For this review, use the dimensioned drawing (mm, ordinates from the lowest corner) and the shaded views. A direction names the side the tool comes from. Give positions to 0.01 mm unless a question says otherwise; leave off trailing zeros. Write each loop counter-clockwise with the first axis right and the second up, starting at its lowest first coordinate (ties: lowest second). Pieces come first, ordered by that corner, then holes. Notation, with made-up numbers: (61.5, 20.5) -> (70.5, 20.5) arc R22 cw to (70.5, 46.5) -> close; hole circle Ø11 at (-10.5, -32). An arc over 180 degrees is marked (long way). Answer as CSV lines item,"result".
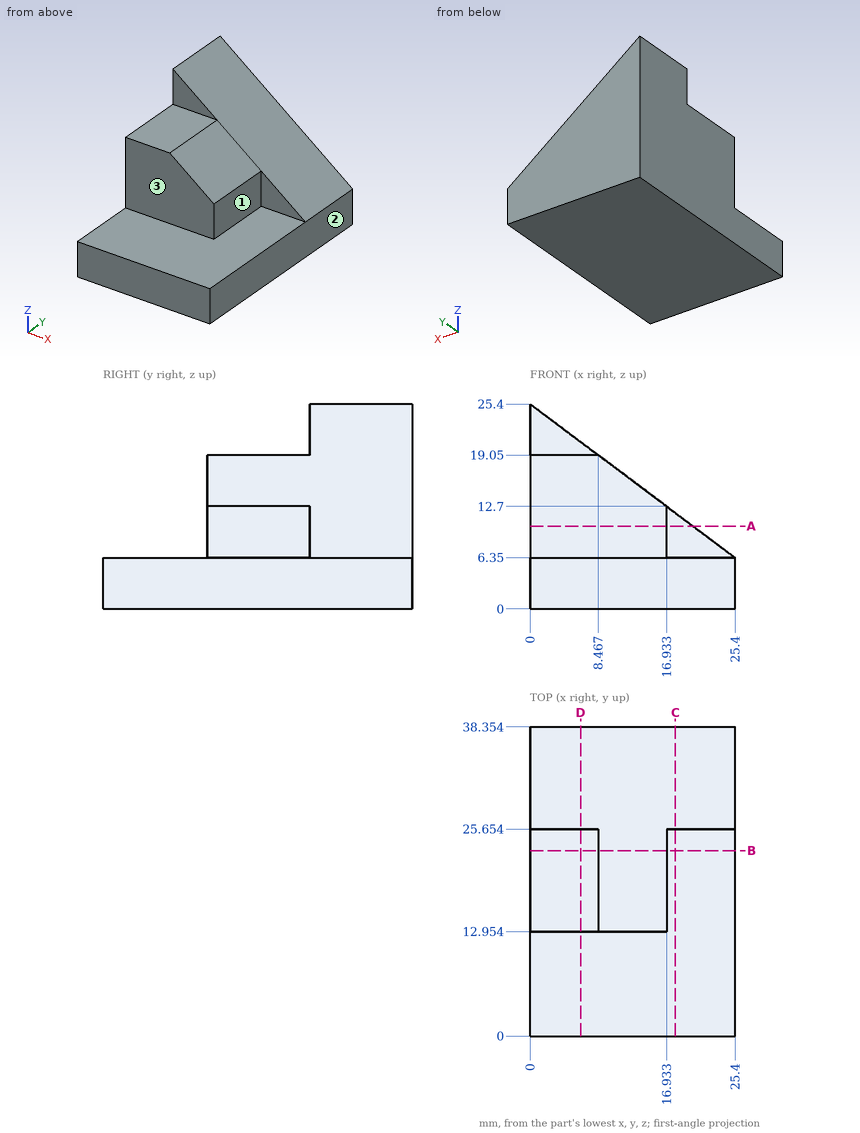
Q1. Add section A-A (z = 10.25). Write out the cut boundary in (x, y), plus the area to 3 significant figures.
Answer block:
outline,"(0, 12.95) -> (16.93, 12.95) -> (16.93, 25.65) -> (20.2, 25.65) -> (20.2, 38.35) -> (0, 38.35) -> close"
area,"472 mm2"
Q2. Add section B-B (y = 23). Write out the cut boundary in (x, z).
Answer block:
outline,"(0, 0) -> (25.4, 0) -> (25.4, 6.35) -> (16.93, 6.35) -> (16.93, 12.7) -> (8.47, 19.05) -> (0, 19.05) -> close"
Q3. To check wall thickness, follow probe 1 along Z at (x, y) = (15.75, 11.5); probe 2 along Y at (x, z) = (1, 23.5); probe 3 along Y at (x, z) = (4.25, 6.5). State the ranges of each line that lie inside material, in increasing order. Write a range as [from, to].
Answer block:
probe 1,"z = [0, 6.35]"
probe 2,"y = [25.65, 38.35]"
probe 3,"y = [12.95, 38.35]"
Q4. For the marked faces 1, 2 and 3, list the 3-axis set-ups (+Z, -Z, +X, -X, +Y, -Y) from which the entire face can be reached by the end or side of a thin tool; tool diameter is ignored.
Answer block:
face 1,"+Z, +X, -Y"
face 2,"+Z, -Z, +X, +Y, -Y"
face 3,"+Z, +X, -X, -Y"
Q5. Clearance check with flat-ended pins moving along their axes: pin 1 (10 mm diameter, centred on x = 4.5, z = 10.5, fed in from -Y); pin 2 (7.5 mm diameter, centred on x = 7.5, y = 11, fed in from +Z); pin 3 (12 mm diameter, centred on x = 15.5, y = 9.5, fed in from +Z) (1 decimal); pin 4 (3 mm diameter, centred on x = 11, y = 20.5, fed in from +Z) (1 decimal). State where each tip first meets the part, or that it passes through.
Answer block:
pin 1,"stops at y = 0"
pin 2,"stops at z = 19.05"
pin 3,"stops at z = 17.5"
pin 4,"stops at z = 18.3"
Q6. Add section D-D (x = 6.25). Write out the cut boundary in (y, z), plus the area to 3 significant figures.
Answer block:
outline,"(0, 0) -> (38.35, 0) -> (38.35, 20.71) -> (25.65, 20.71) -> (25.65, 19.05) -> (12.95, 19.05) -> (12.95, 6.35) -> (0, 6.35) -> close"
area,"587 mm2"
Q7. Add section C-C (x = 18). Write out the cut boundary in (y, z), plus the area to 3 significant figures.
Answer block:
outline,"(0, 0) -> (38.35, 0) -> (38.35, 11.9) -> (25.65, 11.9) -> (25.65, 6.35) -> (0, 6.35) -> close"
area,"314 mm2"
